from build123d import *
from build123d.topology import SkipClean

# Parameters (mm, degrees)
SKIZZE1_R                       = 11
SKIZZE1_R_2                     = 9
AUFSATZ_LINEAR_AUSTRAGEN1_DEPTH = 11
AUFSATZ_LINEAR_START            = 5.5
SKIZZE2_R                       = 9
AUFSATZ_LINEAR_AUSTRAGEN2_DEPTH = 5.5
AUFSATZ_LINEAR_START_2          = 11
SKIZZE3_R                       = 11.75
SKIZZE3_R_2                     = 9
AUFSATZ_LINEAR_AUSTRAGEN3_DEPTH = 11
SKIZZE4_R                       = 10.75
SKIZZE4_R_2                     = 7
AUFSATZ_LINEAR_AUSTRAGEN4_DEPTH = 10


with BuildPart() as part:
    # Skizze1 → Aufsatz-Linear austragen1 (new body)
    with BuildSketch(Plane(origin=(0, 0, 0), x_dir=(1, 0, 0), z_dir=(0, 1, 0))):
        with Locations(Location((0, 0, 0), (0, 0, 270))):
            Circle(SKIZZE1_R)
        with Locations(Location((0, 0, 0), (0, 0, 270))):
            Circle(SKIZZE1_R_2, mode=Mode.SUBTRACT)
    extrude(amount=AUFSATZ_LINEAR_AUSTRAGEN1_DEPTH)

    # Skizze2 → Aufsatz-Linear austragen2 (add)
    with SkipClean():  # the faces are left unmerged after this step: merging them gives an invalid solid
        with BuildSketch(Plane.XZ.offset(AUFSATZ_LINEAR_START)):
            Polygon((15.588457268, 0), (7.794228634, 13.5), (-7.794228634, 13.5), (-15.588457268, 0), (-7.794228634, -13.5), (7.794228634, -13.5), align=None)
            with Locations(Location((0, 0, 0), (0, 0, 270))):
                Circle(SKIZZE2_R, mode=Mode.SUBTRACT)
        extrude(amount=-AUFSATZ_LINEAR_AUSTRAGEN2_DEPTH)

    # Skizze3 → Aufsatz-Linear austragen3 (add)
    with SkipClean():  # the faces are left unmerged after this step: merging them gives an invalid solid
        with BuildSketch(Plane.XZ.offset(5.5).offset(AUFSATZ_LINEAR_START_2)):
            with Locations(Location((0, 0, 0), (0, 0, 270))):
                Circle(SKIZZE3_R)
            with Locations(Location((0, 0, 0), (0, 0, 270))):
                Circle(SKIZZE3_R_2, mode=Mode.SUBTRACT)
        extrude(amount=-AUFSATZ_LINEAR_AUSTRAGEN3_DEPTH)

    # Skizze4 → Aufsatz-Linear austragen4 (add)
    with SkipClean():  # the faces are left unmerged after this step: merging them gives an invalid solid
        with BuildSketch(Plane.XZ.offset(16.5)):
            with Locations(Location((0, 0, 0), (0, 0, 270))):
                Circle(SKIZZE4_R)
            with Locations(Location((0, 0, 0), (0, 0, 270))):
                Circle(SKIZZE4_R_2, mode=Mode.SUBTRACT)
        extrude(amount=AUFSATZ_LINEAR_AUSTRAGEN4_DEPTH)


solid = part.part
Geometry: final body of the model. Coordinates: model frame, mm. A direction names the side the tool comes from. Round coordinates to 2 decimals unless told otherwise and drop trailing zeros. Order: outer loops, then holes, each group sorted by start corner. A loop starts at its lowest first (then second) coordinate and runs counter-clockwise, first axis right, second up. Notation, with made-up numbers: (80.5, 86.25) - (95.5, 86.25) arc R29 ccw to (95.5, 112.25) - close; hole circle Ø1 at (45.25, 46.5). An arc over 180 degrees is marked (long way). Write each question's results on one line, items separated by ' | '.
Item 1: Section D-D, the plane x = 13. Return the cut outline in (y, z), and give its area (3 significant figures).
Completed:
outline: (-5.5, -4.48) - (0, -4.48) - (0, 4.48) - (-5.5, 4.48) - close | area: 49.3 mm^2
Item 2: Section B-B, the plane z = -0.5. Return the cut outline in (x, y).
Completed:
outline: (-15.3, -5.5) - (-11.74, -5.5) - (-11.74, -16.5) - (-10.74, -16.5) - (-10.74, -26.5) - (-6.98, -26.5) - (-6.98, -16.5) - (-8.99, -16.5) - (-8.99, 11) - (-10.99, 11) - (-10.99, 0) - (-15.3, 0) - close; (6.98, -26.5) - (10.74, -26.5) - (10.74, -16.5) - (11.74, -16.5) - (11.74, -5.5) - (15.3, -5.5) - (15.3, 0) - (10.99, 0) - (10.99, 11) - (8.99, 11) - (8.99, -16.5) - (6.98, -16.5) - close
Item 3: Section C-C, the plane y = -11. Return the cut outline in (x, z), and give its area (3 significant figures).
Completed:
outline: circle Ø23.5 at (0, 0); hole circle Ø18 at (0, 0) | area: 179 mm^2
Item 4: Section A-A, the plane x = 0. Return the cut outline in (y, z), and give its area (3 significant figures).
Completed:
outline: (-26.5, -10.75) - (-16.5, -10.75) - (-16.5, -11.75) - (-5.5, -11.75) - (-5.5, -13.5) - (0, -13.5) - (0, -11) - (11, -11) - (11, -9) - (-16.5, -9) - (-16.5, -7) - (-26.5, -7) - close; (-26.5, 7) - (-16.5, 7) - (-16.5, 9) - (11, 9) - (11, 11) - (0, 11) - (0, 13.5) - (-5.5, 13.5) - (-5.5, 11.75) - (-16.5, 11.75) - (-16.5, 10.75) - (-26.5, 10.75) - close | area: 229 mm^2
Item 5: Mould query, pull axis X, two halves, no side actions, for faces 1 (the flat face through (-11.746, -2.788, -6.656)), 2 (the cylindrical face through (-10.74, 5.42, -2.38)), 3 (the flat face through (-7.3, -16.5, 0)), 4 (the cylindrical face through (-6.834, -21.43, 1.517)). Classes: pulls with the +X half, pulls with the -X half, needs draft (parallel to the pull), parting line crosses it, or undercut.
Completed:
face 1: pulls with the -X half | face 2: parting line crosses it | face 3: undercut | face 4: undercut
Item 6: First-contact query: pin 1 Ø11 at (x, z) = (0, 0) entering from -Y; pin 2 Ø8 at (y, z) = (-8.5, 8.5) entering from -X; pin 3 Ø1 at (y, z) = (-10.5, -0.5) entering from -X; pin 4 Ø3 at (x, y) = (-5.5, -21) entering from -Z. Flat tips, straight axial feed; report the tip coordinate or a pass-through.
Completed:
pin 1: through | pin 2: x = -12.21 | pin 3: x = -11.75 | pin 4: z = -9.98
Item 7: Material intervals for line 1 along X through (y, z) = (-13.75, 0); line 2 along Z through (x, y) = (0, -2); line 3 along X through (y, z) = (-21.5, 0), sorted ascending. Write a range as [from, to].
Completed:
line 1: [-11.75, -9], [9, 11.75] | line 2: [-13.5, -9], [9, 13.5] | line 3: [-10.75, -7], [7, 10.75]
Item 8: Reachability of faces 5 (the flat face through (11.5, -5.5, 3.1)), 6 (the flat face through (8, 0, -8)), 7 (the flat face through (-7, -26.5, -2)) from +Z, -Z, +X, -X, +Y, -Y: full face, straight path, thin tool, end or side. Return the list, or none.
Completed:
face 5: -Y | face 6: +Y | face 7: +Z, -Z, +X, -X, -Y
